```python
from build123d import *

# Parameters (mm, degrees)
F1_DEPTH = 12
F3_D     = 5
F3_DEPTH = 20
F3_TIP   = 1.5021515476


with BuildPart() as f1:
    # F0 (on Front) → F1 (new body)
    with BuildSketch(Plane.XZ):
        with BuildLine():
            Line((12, -47), (70, -47))
            Line((70, -47), (70, 47))
            Line((70, 47), (-70, 47))
            Line((-70, 47), (-70, 31.9666295471))
            ThreePointArc((-70, 31.9666295471), (-56, 17), (-70, 2.0333704529))
            Line((-70, 2.0333704529), (-70, -13))
            Line((-70, -13), (12, -13))
            Line((12, -13), (12, -47))
        make_face()
    extrude(amount=F1_DEPTH)

    # F3
    with Locations(Plane(origin=(-70, 0, 0), x_dir=(0, -1, 0), z_dir=(-1, 0, 0))):
        with Locations((6, 40), (6, -6)):
            Hole(F3_D / 2, depth=F3_DEPTH)
            with Locations((0, 0, -(F3_DEPTH + F3_TIP / 2))):  # 118° drill point
                Cone(0, F3_D / 2, F3_TIP, mode=Mode.SUBTRACT)


solid = f1.part
```
The model under review builds one solid part; all positions refer to its coordinate system, in mm. A direction names the side the tool comes from. Round coordinates to 2 decimals unless told otherwise and drop trailing zeros. Write each loop counter-clockwise with the first axis right and the second up, starting at its lowest first coordinate (ties: lowest second). Pieces come first, ordered by that corner, then holes. Notation, with made-up numbers: (59, 65.25) - (112, 65.25) arc R23 ccw to (112, 97.25) - close; hole circle Ø4 at (16.25, 46.5). An arc over 180 degrees is marked (long way). One line per question, with ' | ' between items.
Item 1: Add section B-B, the plane z = -37.5. Give the boundary of the cut face in (x, y), then the cut area to 3 significant figures.
Resolved:
outline: (12, -12) - (70, -12) - (70, 0) - (12, 0) - close | area: 696 mm2
Item 2: To check wall thickness, follow probe 1 along Z at (x, y) = (-55, -6); probe 2 along Y at (x, z) = (-55, 40); probe 3 along Z at (x, y) = (-62.75, -6). State the ranges of each line that lie inside material, in increasing order.
Resolved:
probe 1: z = -13 to -8.5, -3.5 to 37.5, 42.5 to 47 | probe 2: y = -12 to -8.5, -3.5 to 0 | probe 3: z = -13 to -8.5, -3.5 to 4.47, 29.53 to 37.5, 42.5 to 47
Item 3: Add section C-C, the plane x = -3. Give the boundary of the cut face in (y, z).
Resolved:
outline: (-12, -13) - (0, -13) - (0, 47) - (-12, 47) - close
Item 4: For faces 5 (the face through (-59.86, -3.615, -5.249)), 6 (the face through (12, -6, -30)), 7 (the face through (-70, -3, 40)), list the 3-axis set-ups (+Z, -Z, +X, -X, +Y, -Y) from which the entire face can be reached by the end or side of a thin tool; tool diameter is ignored.
Resolved:
face 5: -X | face 6: -Z, -X, +Y, -Y | face 7: +Z, -Z, -X, +Y, -Y
Item 5: The part is to be moulded in two halves that separate along Y. For faces 1 (the face through (15, -12, 11)), 2 (the face through (-48.759, -5.566, -5.981)), 3 (the face through (15, 0, 11)), 4 (the face through (41, -6, -47)), say which applies: pulls with the +Y half, pulls with the -Y half, needs draft (parallel to the pull), parting line crosses it, or undercut.
Resolved:
face 1: pulls with the -Y half | face 2: undercut | face 3: pulls with the +Y half | face 4: needs draft
Item 6: Add section A-A, the plane y = -10.25. Give the boundary of the cut face in (x, z).
Resolved:
outline: (-70, -13) - (12, -13) - (12, -47) - (70, -47) - (70, 47) - (-70, 47) - (-70, 31.97) arc R15 cw to (-70, 2.03) - close
Item 7: For P1, Ø6, axis at y = -3.5, z = -38, coming from the -X side; P2, Ø3, axis at y = -6, z = 40, coming from the -X side; P3, Ø6, axis at y = -6.5, z = 24, coming from the -X side, all flat-tipped, find the tip position at first contact; note any pin that passes through.
Resolved:
P1: stops at x = 12 | P2: stops at x = -49.4 | P3: stops at x = -59.82
